CAD build for the part. Positions are in the model's coordinates, mm. A direction names the side the tool comes from. Round coordinates to 2 decimals unless told otherwise and drop trailing zeros. Write each loop counter-clockwise with the first axis right and the second up, starting at its lowest first coordinate (ties: lowest second). Pieces come first, ordered by that corner, then holes. Notation, with made-up numbers: (39.25, 73.25) - (50.25, 73.25) arc R30 cw to (50.25, 106.25) - close; hole circle Ø9 at (-37, 87.25). An arc over 180 degrees is marked (long way). Answer in a Markdown table with one row per item.
```python
from build123d import *

# Parameters (mm, degrees)
F1_DEPTH      = 38.1
F1_DEPTH_BACK = 38.1
F2_W          = 34.983035177
F2_H          = 57.6349133626
F3_DEPTH      = 14.047474361
F3_DEPTH_BACK = 25.4
F4_R          = 20.8399152663
F5_DEPTH      = 25.4
F6_DEPTH      = 38.1
F6_DEPTH_BACK = 38.1
F7_R          = 8.3166578591
F7_R_2        = 7.3771783421
F8_DEPTH      = 38.101
F8_DEPTH_BACK = 38.101


with BuildPart() as f1:
    # F0 (on Front) → F1 (new body, two sides)
    with BuildSketch(Plane.XZ) as f1_sk:
        with BuildLine():
            ThreePointArc((14.0431994365, 50.8973942286), (14.045655606, 51.0490359422), (14.046474361, 51.2006953359))
            ThreePointArc((14.046474361, 51.2006953359), (-0.0285058427, 65.247140772), (-14.0463586618, 51.1436837678))
            Line((-14.0463586618, 51.1436837678), (14.0431994365, 50.8973942286))
        make_face()
        with BuildLine():
            Line((14.0431994365, 50.8973942286), (-14.0463586618, 51.1436837678))
            ThreePointArc((-14.0463586618, 51.1436837678), (-0.1231549002, 37.1547608762), (14.0431994365, 50.8973942286))
        make_face()
        with BuildLine():
            ThreePointArc((14.0431994365, 50.8973942286), (-0.1231549002, 37.1547608762), (-14.0463586618, 51.1436837678))
            Line((-14.0463586618, 51.1436837678), (-13.7860988001, -12.9784494638))
            Line((-13.7860988001, -12.9784494638), (14.0431994365, -12.9784494638))
            Line((14.0431994365, -12.9784494638), (14.0431994365, 50.8973942286))
        make_face()
    extrude(amount=F1_DEPTH)
    extrude(f1_sk.sketch, amount=-F1_DEPTH_BACK)

    # F2 (on Right) → F3 (cut, two sides)
    with BuildSketch(Plane.YZ) as f3_sk:
        with Locations((0.7638838142, 41.7796033435)):
            Rectangle(F2_W, F2_H)
    extrude(amount=-F3_DEPTH, mode=Mode.SUBTRACT)
    extrude(f3_sk.sketch, amount=F3_DEPTH_BACK, mode=Mode.SUBTRACT)

    # F4 (on Front) → F5 (join)
    with BuildSketch(Plane.XZ):
        Circle(F4_R)
    extrude(amount=F5_DEPTH)

    # F4 (on Front) → F6 (join, two sides)
    with BuildSketch(Plane.XZ) as f6_sk:
        Circle(F4_R)
    extrude(amount=F6_DEPTH)
    extrude(f6_sk.sketch, amount=-F6_DEPTH_BACK)

    # F7 (on Front) → F8 (cut, two sides)
    with BuildSketch(Plane.XZ) as f8_sk:
        Circle(F7_R)
        with Locations((0, 51.9042946398)):
            Circle(F7_R_2)
    extrude(amount=-F8_DEPTH, mode=Mode.SUBTRACT)
    extrude(f8_sk.sketch, amount=F8_DEPTH_BACK, mode=Mode.SUBTRACT)


solid = f1.part
```
Q1. Saw through at A-A on z = 0. List the corners of the cut face in (x, y), then the cut area to 3 significant figures.
Computed:
| item | result |
|---|---|
| outline | (-20.84, -38.1) - (-8.32, -38.1) - (-8.32, 38.1) - (-20.84, 38.1) - close; (8.32, -38.1) - (20.84, -38.1) - (20.84, 38.1) - (8.32, 38.1) - close |
| area | 1,910 mm2 |
Q2. Saw through at D-D on z = 27. List the corners of the cut face in (x, y).
Computed:
| item | result |
|---|---|
| outline | (-13.95, -38.1) - (14.04, -38.1) - (14.04, -16.73) - (-13.95, -16.73) - close; (-13.95, 18.26) - (14.04, 18.26) - (14.04, 38.1) - (-13.95, 38.1) - close |
Q3. Saw through at B-B on x = 0. List the corners of the cut face in (y, z).
Computed:
| item | result |
|---|---|
| outline | (-38.1, -20.84) - (38.1, -20.84) - (38.1, -8.32) - (-38.1, -8.32) - close; (-38.1, 8.32) - (38.1, 8.32) - (38.1, 44.53) - (18.26, 44.53) - (18.26, 20.84) - (-16.73, 20.84) - (-16.73, 44.53) - (-38.1, 44.53) - close; (-38.1, 59.28) - (-16.73, 59.28) - (-16.73, 65.25) - (-38.1, 65.25) - close; (18.26, 59.28) - (38.1, 59.28) - (38.1, 65.25) - (18.26, 65.25) - close |
Q4. Saw through at C-C on y = -14.5. List the corners of the cut face in (x, z), then the cut area to 3 significant figures.
Computed:
| item | result |
|---|---|
| outline | circle Ø41.68 at (0, 0); hole circle Ø16.63 at (0, 0) |
| area | 1,150 mm2 |
Q5. Drill centre lines: line 1 (Z direction, x = 0, y = 29); line 2 (Y direction, x = -8, z = 23); line 3 (Z direction, x = -5.5, y = -26.5). Where is each one in solid material? Low to high.
Computed:
| item | result |
|---|---|
| line 1 | z = -20.84 to -8.32, 8.32 to 44.53, 59.28 to 65.25 |
| line 2 | y = -38.1 to -16.73, 18.26 to 38.1 |
| line 3 | z = -20.1 to -6.24, 6.24 to 46.99, 56.82 to 64.13 |
Q6. 3-axis set-ups, long thin cutter, end or side, ignore diameter. For faces 1 (the cylindrical face through (-0.96, -27.26, 59.22)), 2 (the flat face through (14.043, -28, 33)): which of +Z, -Z, +X, -X, +Y, -Y reach the whole face in a straight line?
Computed:
| item | result |
|---|---|
| face 1 | +Y, -Y |
| face 2 | +Z, +X, +Y, -Y |
Q7. Pull direction Y, two halves, no side cores. Call faces 3 (the flat face through (0, 18.255, 40)), 4 (the flat face through (0, 38.1, 23)), 5 (the flat face through (14.043, 28, 33)): released by +Y, released by -Y, zero draft, split by the parting line, or undercut.
Computed:
| item | result |
|---|---|
| face 3 | undercut |
| face 4 | released by +Y |
| face 5 | zero draft |
Q8. Flat gauge pins, fed straight in: pin 1 (3 mm diameter, centred on y = -23, z = -11, fed in from -X); pin 2 (16 mm diameter, centred on y = 29.5, z = 40.5, fed in from +X); pin 3 (1.5 mm diameter, centred on x = -8.5, y = -29, fed in from -Z). Where does each tip first touch, or does it go through?
Computed:
| item | result |
|---|---|
| pin 1 | stops at x = -18.55 |
| pin 2 | stops at x = 14.04 |
| pin 3 | stops at z = -19.35 |
